Design review of the part shown in the three views and the two pictorial views. Dimensions are in mm from the part's minimum x, y and z. A direction names the side the tool comes from. Coordinates: 2 decimals unless noted, no trailing zeros. Loops run counter-clockwise (first coordinate to the right, second up) from the corner with the lowest first, then second, coordinate; pieces in that order, holes last. Notation, with made-up numbers: (-25, -26) -> (8, -26) arc R14 ccw to (8, -11) -> close; hole circle Ø2 at (-27.5, 35). An arc over 180 degrees is marked (long way). Answer in a Markdown table with one row per item.
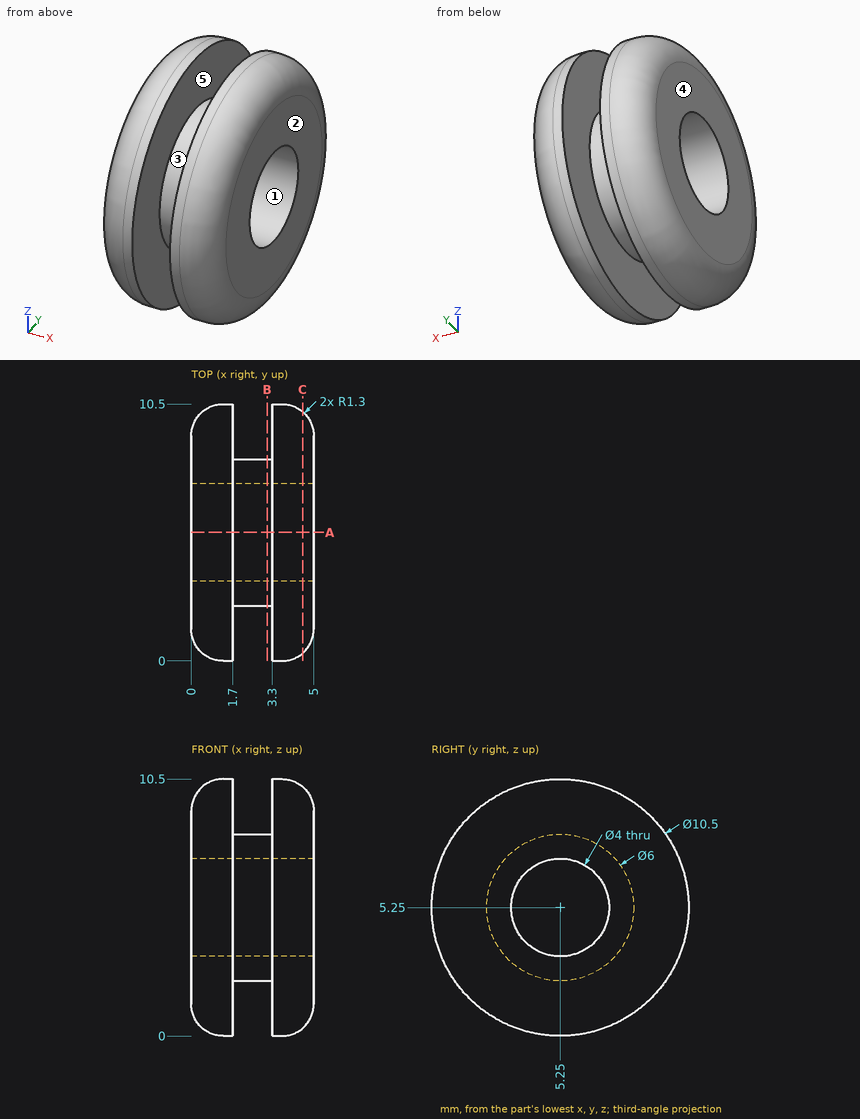
(1) For pin 1 (1.5 mm diameter, centred on x = 2, z = 6, fed in from -Y); pin 2 (1 mm diameter, centred on x = 4, y = 2, fed in from +Z); pin 3 (2 mm diameter, centred on x = 2.5, z = 7.5, fed in from +Y); pin 4 (3 mm diameter, centred on x = 4, z = 2, fed in from -Y), all flat-tipped, find the tip position at first contact; note any pin that passes through.
Evaluation:
| item | result |
|---|---|
| pin 1 | stops at y = 0 |
| pin 2 | stops at z = 9.7 |
| pin 3 | stops at y = 10.23 |
| pin 4 | stops at y = 0.31 |
(2) Take a section at B-B on x = 3.1. Give the boundary of the cut face in (y, z), and give its area (3 significant figures).
Evaluation:
| item | result |
|---|---|
| outline | circle Ø6 at (5.25, 5.25); hole circle Ø4 at (5.25, 5.25) |
| area | 15.7 mm² |
(3) Take a section at C-C on x = 4.55. Give the boundary of the cut face in (y, z).
Evaluation:
| item | result |
|---|---|
| outline | circle Ø9.87 at (5.25, 5.25); hole circle Ø4 at (5.25, 5.25) |
(4) Take a section at A-A on y = 5.25. Give the boundary of the cut face in (x, z).
Evaluation:
| item | result |
|---|---|
| outline | (0, 1.3) arc R1.3 ccw to (1.3, 0) -> (1.7, 0) -> (1.7, 2.25) -> (3.3, 2.25) -> (3.3, 0) -> (3.7, 0) arc R1.3 ccw to (5, 1.3) -> (5, 3.25) -> (0, 3.25) -> close; (0, 7.25) -> (5, 7.25) -> (5, 9.2) arc R1.3 ccw to (3.7, 10.5) -> (3.3, 10.5) -> (3.3, 8.25) -> (1.7, 8.25) -> (1.7, 10.5) -> (1.3, 10.5) arc R1.3 ccw to (0, 9.2) -> close |
(5) Tool access review of the marked faces 4 and 5: name each direction out of +Z, -Z, +X, -X, +Y, -Y from which nothing blocks a thin tool from reaching the whole face with its end or side.
Evaluation:
| item | result |
|---|---|
| face 4 | +Z, -Z, -X, +Y, -Y |
| face 5 | none |
(6) Draft analysis for pull direction Y (two halves, no side actions). For the marked faces 1, 2 and 3, state which applies: pulls with the +Y half, pulls with the -Y half, needs draft (parallel to the pull), parting line crosses it, or undercut.
Evaluation:
| item | result |
|---|---|
| face 1 | undercut |
| face 2 | needs draft |
| face 3 | parting line crosses it |
(7) To check wall thickness, follow probe 1 along Z at (x, y) = (3, 5.25); probe 2 along X at (y, z) = (3.75, 8.75); probe 3 along Z at (x, y) = (3.5, 5.25). State the ranges of each line that lie inside material, in increasing order.
Evaluation:
| item | result |
|---|---|
| probe 1 | z = 2.25 to 3.25, 7.25 to 8.25 |
| probe 2 | x = 0 to 1.7, 3.3 to 5 |
| probe 3 | z = 0 to 3.25, 7.25 to 10.5 |
